```python
from build123d import *

# Parameters (mm, degrees)
SKETCH_1_R          = 13.5
EXTRUDE_1_DEPTH     = 2.8
SKETCH_2_R          = 13
CUT_EXTRUDE_1_DEPTH = 1
SKETCH_5_R          = 11
CUT_EXTRUDE_2_DEPTH = 0.6
CUT_EXTRUDE_3_DEPTH = 0.7
EXTRUDE_2_DEPTH     = 2.8
FILLET_1_R          = 0.2


with BuildPart() as part:
    # 草图1 → 凸台-拉伸1 (new body)
    with BuildSketch(Plane(origin=(0, 0, 0), x_dir=(1, 0, 0), z_dir=(0, 1, 0))):
        with Locations(Location((0, 0, 0), (0, 0, 270))):
            Circle(SKETCH_1_R)
    extrude(amount=EXTRUDE_1_DEPTH)

    # 草图2 → 切除-拉伸1 (cut)
    with BuildSketch(Plane(origin=(0, 2.8, 0), x_dir=(1, 0, 0), z_dir=(0, 1, 0))):
        with Locations(Location((0, 0, 0), (0, 0, 270))):
            Circle(SKETCH_2_R)
    extrude(amount=-CUT_EXTRUDE_1_DEPTH, mode=Mode.SUBTRACT)

    # 草图4 → 切除-旋转1 (revolve, cut)
    with BuildSketch(Plane.XY):
        Polygon((0, 1.3), (-11, 1.3), (-13, 1.8), (0, 1.8), align=None)
    revolve(axis=Axis((0, 1.8, 0), (0, -1, 0)), mode=Mode.SUBTRACT)

    # 草图5 → 切除-拉伸2 (cut)
    with BuildSketch(Plane(origin=(0, 1.3, 0), x_dir=(1, 0, 0), z_dir=(0, 1, 0))):
        with Locations(Location((0, 0, 0), (0, 0, 180))):
            Circle(SKETCH_5_R)
    extrude(amount=-CUT_EXTRUDE_2_DEPTH, mode=Mode.SUBTRACT)

    # 草图6 → 切除-拉伸3 (cut)
    with BuildSketch(Plane(origin=(0, 0.7, 0), x_dir=(1, 0, 0), z_dir=(0, 1, 0))):
        with BuildLine():
            ThreePointArc((-3.539967162, 9.352466653), (-3.826834324, 9.238795325), (-4.110057805, 9.116327377))
            ThreePointArc((-4.110057805, 9.116327377), (-5.5, 9.526279442), (-5.839942195, 8.117578159))
            ThreePointArc((-5.839942195, 8.117578159), (-6.08761429, 7.933533403), (-6.329490128, 7.741934817))
            ThreePointArc((-6.329490128, 7.741934817), (-7.778174593, 7.778174593), (-7.741934817, 6.329490128))
            ThreePointArc((-7.741934817, 6.329490128), (-7.933533403, 6.08761429), (-8.117578159, 5.839942195))
            ThreePointArc((-8.117578159, 5.839942195), (-9.526279442, 5.5), (-9.116327377, 4.110057805))
            ThreePointArc((-9.116327377, 4.110057805), (-9.238795325, 3.826834324), (-9.352466653, 3.539967162))
            ThreePointArc((-9.352466653, 3.539967162), (-10.137444482, 3.466448921), (-10.625184089, 2.847009496))
            ThreePointArc((-10.625184089, 2.847009496), (-11, 0), (-10.625184089, -2.847009496))
            ThreePointArc((-10.625184089, -2.847009496), (-10.137444482, -3.466448921), (-9.352466653, -3.539967162))
            ThreePointArc((-9.352466653, -3.539967162), (-9.238795325, -3.826834324), (-9.116327377, -4.110057805))
            ThreePointArc((-9.116327377, -4.110057805), (-9.526279442, -5.5), (-8.117578159, -5.839942195))
            ThreePointArc((-8.117578159, -5.839942195), (-7.933533403, -6.08761429), (-7.741934817, -6.329490128))
            ThreePointArc((-7.741934817, -6.329490128), (-7.778174593, -7.778174593), (-6.329490128, -7.741934817))
            ThreePointArc((-6.329490128, -7.741934817), (-6.08761429, -7.933533403), (-5.839942195, -8.117578159))
            ThreePointArc((-5.839942195, -8.117578159), (-5.5, -9.526279442), (-4.110057805, -9.116327377))
            ThreePointArc((-4.110057805, -9.116327377), (-3.826834324, -9.238795325), (-3.539967162, -9.352466653))
            ThreePointArc((-3.539967162, -9.352466653), (-3.466448921, -10.137444482), (-2.847009496, -10.625184089))
            ThreePointArc((-2.847009496, -10.625184089), (0, -11), (2.847009496, -10.625184089))
            ThreePointArc((2.847009496, -10.625184089), (3.466448921, -10.137444482), (3.539967162, -9.352466653))
            ThreePointArc((3.539967162, -9.352466653), (3.826834324, -9.238795325), (4.110057805, -9.116327377))
            ThreePointArc((4.110057805, -9.116327377), (5.5, -9.526279442), (5.839942195, -8.117578159))
            ThreePointArc((5.839942195, -8.117578159), (6.08761429, -7.933533403), (6.329490128, -7.741934817))
            ThreePointArc((6.329490128, -7.741934817), (7.778174593, -7.778174593), (7.741934817, -6.329490128))
            ThreePointArc((7.741934817, -6.329490128), (7.933533403, -6.08761429), (8.117578159, -5.839942195))
            ThreePointArc((8.117578159, -5.839942195), (9.526279442, -5.5), (9.116327377, -4.110057805))
            ThreePointArc((9.116327377, -4.110057805), (9.238795325, -3.826834324), (9.352466653, -3.539967162))
            ThreePointArc((9.352466653, -3.539967162), (10.137444482, -3.466448921), (10.625184089, -2.847009496))
            ThreePointArc((10.625184089, -2.847009496), (11, 0), (10.625184089, 2.847009496))
            ThreePointArc((10.625184089, 2.847009496), (10.137444482, 3.466448921), (9.352466653, 3.539967162))
            ThreePointArc((9.352466653, 3.539967162), (9.238795325, 3.826834324), (9.116327377, 4.110057805))
            ThreePointArc((9.116327377, 4.110057805), (9.526279442, 5.5), (8.117578159, 5.839942195))
            ThreePointArc((8.117578159, 5.839942195), (7.933533403, 6.08761429), (7.741934817, 6.329490128))
            ThreePointArc((7.741934817, 6.329490128), (7.778174593, 7.778174593), (6.329490128, 7.741934817))
            ThreePointArc((6.329490128, 7.741934817), (6.08761429, 7.933533403), (5.839942195, 8.117578159))
            ThreePointArc((5.839942195, 8.117578159), (5.5, 9.526279442), (4.110057805, 9.116327377))
            ThreePointArc((4.110057805, 9.116327377), (3.826834324, 9.238795325), (3.539967162, 9.352466653))
            ThreePointArc((3.539967162, 9.352466653), (3.466448921, 10.137444482), (2.847009496, 10.625184089))
            ThreePointArc((2.847009496, 10.625184089), (0, 11), (-2.847009496, 10.625184089))
            ThreePointArc((-2.847009496, 10.625184089), (-3.466448921, 10.137444482), (-3.539967162, 9.352466653))
        make_face()
    extrude(amount=-CUT_EXTRUDE_3_DEPTH, mode=Mode.SUBTRACT)

    # 草图7 → 凸台-拉伸2 (add)
    with BuildSketch(Plane(origin=(0, 0, 0), x_dir=(1, 0, 0), z_dir=(0, 1, 0))):
        with BuildLine():
            ThreePointArc((-17.384313485, -6.327372652), (0, -18.5), (17.384313485, -6.327372652))
            ThreePointArc((17.384313485, -6.327372652), (17.00124382, -2.09192454), (13.496286822, 0.316610185))
            ThreePointArc((13.496286822, 0.316610185), (0, -13.5), (-13.496286822, 0.316610185))
            ThreePointArc((-13.496286822, 0.316610185), (-17.00124382, -2.09192454), (-17.384313485, -6.327372652))
        make_face()
    extrude(amount=EXTRUDE_2_DEPTH)

    # 圆角1
    fillet_1_edges = [part.edges().sort_by_distance(p)[0] for p in [
        (-17.00124382, 2.8, 2.09192454),
        (0, 2.8, 18.5),
        (17.00124382, 2.8, 2.09192454),
        (0, 2.8, -13.5),
    ]]
    fillet(fillet_1_edges, radius=FILLET_1_R)


solid = part.part
```
Can you work these out from the model? Positions are in its coordinate system, mm. A direction names the side the tool comes from. Coordinates: 2 decimals unless noted, no trailing zeros. Loops run counter-clockwise (first coordinate to the right, second up) from the corner with the lowest first, then second, coordinate; pieces in that order, holes last. Notation, with made-up numbers: M -27,28.5 L -4,28.5 A27 cw -4,51.5 Z; hole C -21.5,-35 d2. An arc over 180 degrees is marked long. Put each result on its own line as item: value. Start each with the question number.
(1) I need wall thicknesses on probe 1 along Z at (x, y) = (0, 1.05); probe 2 along Z at (x, y) = (0, 2.5); probe 3 along X at (y, z) = (2.25, 0). Which ranges of each line are inside material? Lowest first, please.
(2) Which directions (+Z, -Z, +X, -X, +Y, -Y) give clear straight access to the entire face, cutting with the end or side of a thin tool? Please do faces 4 (the face through (8.4, 0.7, 6.5)), 5 (the face through (5.48, 0.355, 9.537)).
(3) We'd pull the mould along Z, two halves only. Please class faces 1 (the face through (-1, 2.8, 14)), 2 (the face through (17.032, 1.282, 2.145)), 3 (the face through (6.5, 0.7, -8.5)): +Z half, -Z half, draft (parallel to the pull), parting line (faces both ways), or undercut.
(4) Will these pins go through, and if not, where does the flat tip stop? pin 1 Ø0.8 at (x, z) = (-10, 4.5) entering from +Y; pin 2 Ø1.4 at (x, z) = (-7, 9) entering from +Y; pin 3 Ø1.4 at (x, z) = (-9, -6.5) entering from +Y; pin 4 Ø3 at (x, z) = (-1, -9) entering from +Y.
(5) Imagine slicing it at A-A on x = 0. List the corners of the cut face in (y, z) for me, and give its area (3 significant figures).
Worked answers:
1. probe 1: z = -13.5 to -11, 11 to 18.5
1. probe 2: z = -13.5 to -13, 13 to 18.5
1. probe 3: x = -14.6 to -13, 13 to 14.6
2. face 4: +Y
2. face 5: +Y, -Y
3. face 1: draft
3. face 2: parting line
3. face 3: undercut
4. pin 1: stops at y = 1.39
4. pin 2: stops at y = 1.58
4. pin 3: stops at y = 1.5
4. pin 4: passes through
5. outline: M 0,-13.5 L 2.6,-13.5 A0.2 ccw 2.8,-13.3 L 2.8,-13 L 1.8,-13 L 1.3,-11 L 0,-11 Z; M 0,11 L 1.3,11 L 1.8,13 L 2.8,13 L 2.8,18.3 A0.2 ccw 2.6,18.5 L 0,18.5 Z
5. area: 23.0 mm2
